Study the drawing (mm; zero at the part's minimum x, y, z) and answer. Round coordinates to 2 decimals unless told otherwise and drop trailing zeros. Write each loop counter-clockwise with the first axis right and the second up, starting at its lowest first coordinate (ties: lowest second). Pieces come first, ordered by that corner, then holes. Notation, with made-up numbers: (77.25, 49.5) - (111.25, 49.5) arc R14 cw to (111.25, 75.5) - close; hole circle Ø9 at (-34.75, 3). An arc over 180 degrees is marked (long way). Return JSON: item names as keys, results as strings. Group by question number.
(1) Section A-A, the plane y = 10 is taken. Write down the section's boundary in (x, z).
(2) Section D-D, the plane y = 17.75 is taken. Write down the section's boundary in (x, z), then the cut area to 4 significant figures.
(3) Section B-B, the plane x = 27.5 is taken. Write down the section's boundary in (y, z), then the cut area to 3 significant figures.
(4) Section C-C, the plane z = 1.3 is taken. Write down the section's boundary in (x, y), then the cut area to 3 significant figures.
(5) Determine the mould class of the marked faces 1, 2, 3 and 4 for opening direction X: +X half, -X half, draft (parallel to the pull), parting line (faces both ways), or undercut.
(6) Find the intervals of material crossed by line 1 along Y through (x, z) = (27.5, 2); line 2 along X through (y, z) = (12.25, 2.45); line 3 along X through (y, z) = (11.5, 2.75), in increasing order. Write a range as [from, to].
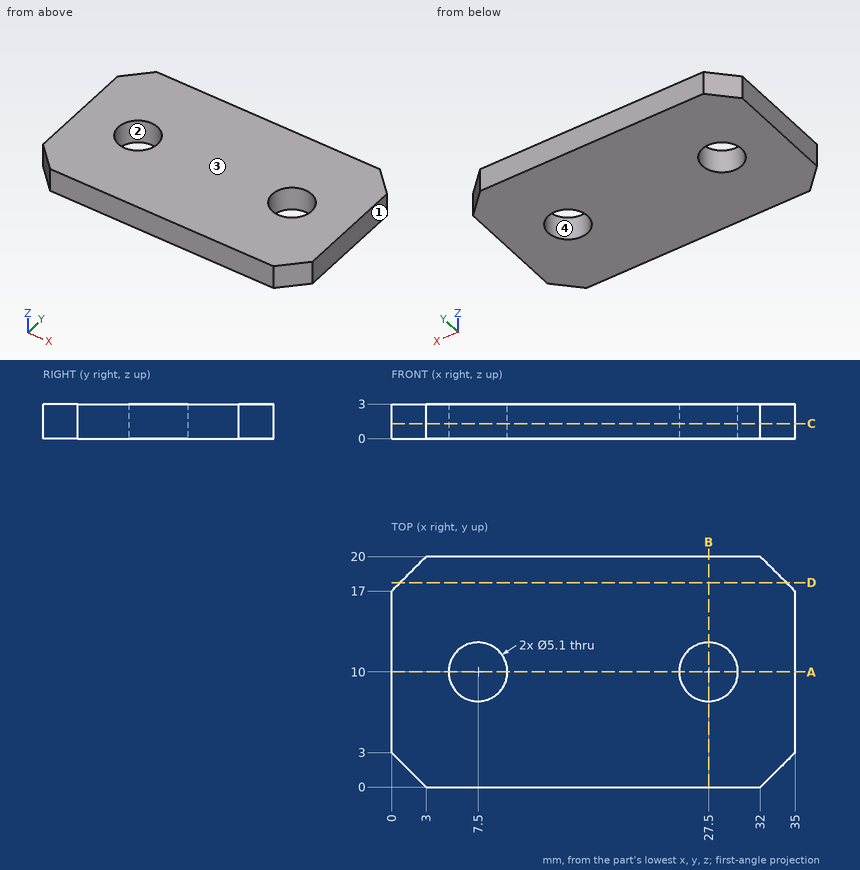
Working result:
{
 "1": {"outline": "(0, 0) - (4.95, 0) - (4.95, 3) - (0, 3) - close; (10.05, 0) - (24.95, 0) - (24.95, 3) - (10.05, 3) - close; (30.05, 0) - (35, 0) - (35, 3) - (30.05, 3) - close"},
 "2": {"outline": "(0.75, 0) - (34.25, 0) - (34.25, 3) - (0.75, 3) - close", "area": "100.5 mm^2"},
 "3": {"outline": "(0, 0) - (7.45, 0) - (7.45, 3) - (0, 3) - close; (12.55, 0) - (20, 0) - (20, 3) - (12.55, 3) - close", "area": "44.7 mm^2"},
 "4": {"outline": "(0, 3) - (3, 0) - (32, 0) - (35, 3) - (35, 17) - (32, 20) - (3, 20) - (0, 17) - close; hole circle Ø5.1 at (7.5, 10); hole circle Ø5.1 at (27.5, 10)", "area": "641 mm^2"},
 "5": {"face 1": "+X half", "face 2": "undercut", "face 3": "draft", "face 4": "undercut"},
 "6": {"line 1": "y = [0, 7.45], [12.55, 20]", "line 2": "x = [0, 6.3], [8.7, 26.3], [28.7, 35]", "line 3": "x = [0, 5.44], [9.56, 25.44], [29.56, 35]"}
}
